```python
from build123d import *

# Parameters (mm, degrees)
F0_R     = 2.375
F0_W     = 26.5
F0_H     = 34.5
F1_DEPTH = 5
F0_W_2   = 22.3
F0_H_2   = 30.5
F2_DEPTH = 2


# Not quite as in the source:
# - a feature of the source that left no trace in its solid (it failed there, or was rolled back) is left out


with BuildPart() as f1:
    # F0 (on Front) → F1 (new body)
    with BuildSketch(Plane.XZ):
        with BuildLine():
            Line((52.45, 19.95), (-52.45, 19.95))
            ThreePointArc((-52.45, 19.95), (-59.5210678119, 17.0210678119), (-62.45, 9.95))
            Line((-62.45, 9.95), (-62.45, -9.95))
            ThreePointArc((-62.45, -9.95), (-59.5210678119, -17.0210678119), (-52.45, -19.95))
            Line((-52.45, -19.95), (52.45, -19.95))
            ThreePointArc((52.45, -19.95), (59.5210678119, -17.0210678119), (62.45, -9.95))
            Line((62.45, -9.95), (62.45, 9.95))
            ThreePointArc((62.45, 9.95), (59.5210678119, 17.0210678119), (52.45, 19.95))
        make_face()
        with Locations((-51.325, 0)):
            Circle(F0_R, mode=Mode.SUBTRACT)
        with Locations((-31, 0)):
            Rectangle(F0_W, F0_H, mode=Mode.SUBTRACT)
        Rectangle(F0_W, F0_H, mode=Mode.SUBTRACT)
        with Locations((31, 0)):
            Rectangle(F0_W, F0_H, mode=Mode.SUBTRACT)
        with Locations((51.325, 0)):
            Circle(F0_R, mode=Mode.SUBTRACT)
    extrude(amount=F1_DEPTH)

    # F0 (on Front) → F2 (join)
    with BuildSketch(Plane.XZ):
        with Locations((-31, 0)):
            Rectangle(F0_W, F0_H)
        with Locations((-31, 0)):
            Rectangle(F0_W_2, F0_H_2, mode=Mode.SUBTRACT)
        Rectangle(F0_W, F0_H)
        Rectangle(F0_W_2, F0_H_2, mode=Mode.SUBTRACT)
        with Locations((31, 0)):
            Rectangle(F0_W, F0_H)
        with Locations((31, 0)):
            Rectangle(F0_W_2, F0_H_2, mode=Mode.SUBTRACT)
    extrude(amount=F2_DEPTH)


solid = f1.part
```
Read the model definition and answer for the solid it produces. Units are mm, in the model's axes. A direction names the side the tool comes from. Round coordinates to 2 decimals unless told otherwise and drop trailing zeros. Write each loop counter-clockwise with the first axis right and the second up, starting at its lowest first coordinate (ties: lowest second). Pieces come first, ordered by that corner, then holes. Notation, with made-up numbers: (27, 43.5) -> (61, 43.5) arc R26 cw to (61, 58.5) -> close; hole circle Ø11 at (67, -27.5). An arc over 180 degrees is marked (long way). Answer in a Markdown table with one row per item. Add a question column.
1) Given P1, Ø8, axis at x = -3.5, z = -2.5, coming from the -Y side; P2, Ø6, axis at x = -41.5, z = 1, coming from the -Y side, each flat-ended and moving along its own axis, determine where each tip first touches the part or whether it passes through.
2) Find section C-C, the plane y = -3. Determine the outline of the cut face in (x, z) (3 decimals).
3) Find section D-D, the plane z = 0. State how many separate pieces and enclosed holes the cut face has, and give its area (3 significant figures).
4) Find section B-B, the plane z = 6.5. Determine the outline of the cut face in (x, y), and give its area (3 significant figures).
5) Which of the six approach directions +Z, -Z, +X, -X, +Y, -Y give full straight-line access (tool end or side, diameter ignored) to faces 4 (the face through (31, -3, -17.25)), 5 (the face through (31, -1, -15.25)), 6 (the face through (-1, -2, -19.95))?
6) Consider line 1 (X direction, y = -1.7, z = 7.5); line 2 (X direction, y = -3.75, z = 3.5); line 3 (Z direction, x = 1, y = -2.25). Determine where each line is inside the solid, lowest interval first.
7) Determine the mould class of faces 1 (the face through (-49.06, -2.46, 0.71)), 2 (the face through (-15, 0, 0)), 3 (the face through (-59.44, -2.46, 17.1)) for opening direction Z: pulls with the +Z half, pulls with the -Z half, needs draft (parallel to the pull), parting line crosses it, or undercut.
8) Find section A-A, the plane x = -28. Determine the outline of the cut face in (y, z).
Findings below:
| question | item | result |
|---|---|---|
| 1 | P1 | through |
| 1 | P2 | y = -5 |
| 2 | outline | (-62.45, -9.95) arc R10 ccw to (-52.45, -19.95) -> (52.45, -19.95) arc R10 ccw to (62.45, -9.95) -> (62.45, 9.95) arc R10 ccw to (52.45, 19.95) -> (-52.45, 19.95) arc R10 ccw to (-62.45, 9.95) -> close; hole circle Ø4.75 at (-51.325, 0); hole (-44.25, -17.25) -> (-17.75, -17.25) -> (-17.75, 17.25) -> (-44.25, 17.25) -> close; hole (-13.25, -17.25) -> (13.25, -17.25) -> (13.25, 17.25) -> (-13.25, 17.25) -> close; hole (17.75, -17.25) -> (44.25, -17.25) -> (44.25, 17.25) -> (17.75, 17.25) -> close; hole circle Ø4.75 at (51.325, 0) |
| 3 | separate pieces | 6 |
| 3 | enclosed holes | 0 |
| 3 | area | 205 mm² |
| 4 | outline | (-62.45, -5) -> (-44.25, -5) -> (-44.25, -2) -> (-42.15, -2) -> (-42.15, 0) -> (-62.45, 0) -> close; (-19.85, -2) -> (-17.75, -2) -> (-17.75, -5) -> (-13.25, -5) -> (-13.25, -2) -> (-11.15, -2) -> (-11.15, 0) -> (-19.85, 0) -> close; (11.15, -2) -> (13.25, -2) -> (13.25, -5) -> (17.75, -5) -> (17.75, -2) -> (19.85, -2) -> (19.85, 0) -> (11.15, 0) -> close; (42.15, -2) -> (44.25, -2) -> (44.25, -5) -> (62.45, -5) -> (62.45, 0) -> (42.15, 0) -> close |
| 4 | area | 252 mm² |
| 5 | face 4 | -Y |
| 5 | face 5 | +Y, -Y |
| 5 | face 6 | -Z, +X, -X, +Y, -Y |
| 6 | line 1 | -62.45 to -42.15, -19.85 to -11.15, 11.15 to 19.85, 42.15 to 62.45 |
| 6 | line 2 | -62.45 to -44.25, -17.75 to -13.25, 13.25 to 17.75, 44.25 to 62.45 |
| 6 | line 3 | -19.95 to -17.25, 17.25 to 19.95 |
| 7 | face 1 | undercut |
| 7 | face 2 | needs draft |
| 7 | face 3 | pulls with the +Z half |
| 8 | outline | (-5, -19.95) -> (0, -19.95) -> (0, -15.25) -> (-2, -15.25) -> (-2, -17.25) -> (-5, -17.25) -> close; (-5, 17.25) -> (-2, 17.25) -> (-2, 15.25) -> (0, 15.25) -> (0, 19.95) -> (-5, 19.95) -> close |
